```python
from build123d import *

# Parameters (mm, degrees)
SKETCH1_W               = 95.25
SKETCH1_H               = 95.25
BOSS_EXTRUDE1_DEPTH     = 6.35
SKETCH4_W               = 6.35
SKETCH4_H               = 95.25
BOSS_EXTRUDE2_DEPTH     = 12.7
CUT_EXTRUDE1_DEPTH      = 102.649597269
CUT_EXTRUDE1_DEPTH_BACK = 102.649597269
SKETCH5_W               = 22.86
SKETCH5_H               = 12.7
SKETCH6_R               = 1.27
CUT_EXTRUDE2_DEPTH      = 108.247345538
SKETCH7_R               = 1.5875
CUT_EXTRUDE3_DEPTH      = 69.538830235
CUT_EXTRUDE4_DEPTH      = 102.649597269
CUT_EXTRUDE4_DEPTH_BACK = 102.649597269
SKETCH8_R               = 1.5875
SKETCH9_W               = 95.25
SKETCH9_H               = 19.05
BOSS_EXTRUDE3_DEPTH     = 3.175
CUT_EXTRUDE5_DEPTH      = 71.781852371
SKETCH11_W              = 50.8
SKETCH11_H              = 38.1
BOSS_EXTRUDE4_DEPTH     = 4.7625
CUT_EXTRUDE6_REACH      = 115.858
SKETCH12_R              = 1.5875
SKETCH12_W              = 19.05
SKETCH12_H              = 15.875
FILLET1_R               = 6.985
FILLET2_R               = 6.35
FILLET3_R               = 3.175
FILLET4_R               = 3.175
FILLET5_R               = 3.175
SKETCH14_W              = 9.525
SKETCH14_H              = 9.525
BOSS_EXTRUDE5_DEPTH     = 9.525
SKETCH15_R              = 1.905
CUT_EXTRUDE7_DEPTH      = 76.268261904
FILLET7_R               = 1.5875
FILLET8_R               = 1.5875
CUT_EXTRUDE8_START      = -3.175
CUT_EXTRUDE8_DEPTH      = 3.175


with BuildPart() as part:
    # Sketch1 → Boss-Extrude1 (new body)
    with BuildSketch(Plane(origin=(0, 0, 0), x_dir=(1, 0, 0), z_dir=(0, 1, 0))):
        Rectangle(SKETCH1_W, SKETCH1_H)
    extrude(amount=BOSS_EXTRUDE1_DEPTH)

    # Sketch4 → Boss-Extrude2 (add)
    with BuildSketch(Plane(origin=(0, 0, 0), x_dir=(-1, 0, 0), z_dir=(0, -1, 0))):
        with Locations((-44.45, 0)):
            Rectangle(SKETCH4_W, SKETCH4_H)
        with Locations((44.45, 0)):
            Rectangle(SKETCH4_W, SKETCH4_H)
    extrude(amount=BOSS_EXTRUDE2_DEPTH)

    # Sketch5 → Cut-Extrude1 (cut, two sides: drawn at the far end of the back side and taken through both)
    with BuildSketch(Plane(origin=(-41.275, 0, 0), x_dir=(0, 0, -1), z_dir=(1, 0, 0)).offset(-CUT_EXTRUDE1_DEPTH_BACK)):
        with Locations((-22.225, -6.35)):
            Rectangle(SKETCH5_W, SKETCH5_H)
    extrude(amount=CUT_EXTRUDE1_DEPTH + CUT_EXTRUDE1_DEPTH_BACK, mode=Mode.SUBTRACT)

    # Sketch6 → Cut-Extrude2 (cut, through all)
    with BuildSketch(Plane.ZY.offset(47.625)):
        with Locations((36.068, -6.35)):
            Circle(SKETCH6_R)
        with Locations((8.382, -6.35)):
            Circle(SKETCH6_R)
    extrude(amount=-CUT_EXTRUDE2_DEPTH, mode=Mode.SUBTRACT)

    # Sketch7 → Cut-Extrude3 (cut, through all)
    with BuildSketch(Plane.XZ):
        with Locations(Location((27.94, 0, 0), (0, 0, 270))):
            Circle(SKETCH7_R)
        with Locations(Location((-27.94, 0, 0), (0, 0, 270))):
            Circle(SKETCH7_R)
        with Locations(Location((0, 36.83, 0), (0, 0, 270))):
            Circle(SKETCH7_R)
        with Locations(Location((0, -36.83, 0), (0, 0, 270))):
            Circle(SKETCH7_R)
    extrude(amount=-CUT_EXTRUDE3_DEPTH, mode=Mode.SUBTRACT)

    # Sketch8 → Cut-Extrude4 (cut, two sides: drawn at the far end of the back side and taken through both)
    with BuildSketch(Plane(origin=(-41.275, 0, 0), x_dir=(0, 0, -1), z_dir=(1, 0, 0)).offset(-CUT_EXTRUDE4_DEPTH_BACK)):
        with Locations((41.275, -6.35)):
            Circle(SKETCH8_R)
        with Locations((33.3375, -6.35)):
            Circle(SKETCH8_R)
    extrude(amount=CUT_EXTRUDE4_DEPTH + CUT_EXTRUDE4_DEPTH_BACK, mode=Mode.SUBTRACT)

    # Sketch9 → Boss-Extrude3 (add)
    with BuildSketch(Plane.XY.offset(47.625)):
        with Locations((0, -3.175)):
            Rectangle(SKETCH9_W, SKETCH9_H)
    extrude(amount=BOSS_EXTRUDE3_DEPTH)

    # Sketch10 → Cut-Extrude5 (cut, through all)
    with BuildSketch(Plane.XZ):
        with BuildLine():
            Line((-31.75, -38.735), (-35.56, -38.735))
            ThreePointArc((-35.56, -38.735), (-37.356051224, -37.991051224), (-38.1, -36.195))
            Line((-38.1, -36.195), (-38.1, -15.875))
            ThreePointArc((-38.1, -15.875), (-37.356051224, -14.078948776), (-35.56, -13.335))
            Line((-35.56, -13.335), (-31.75, -13.335))
            ThreePointArc((-31.75, -13.335), (-29.953948776, -14.078948776), (-29.21, -15.875))
            Line((-29.21, -15.875), (-29.21, -36.195))
            ThreePointArc((-29.21, -36.195), (-29.953948776, -37.991051224), (-31.75, -38.735))
        make_face()
        with BuildLine():
            Line((35.56, -38.735), (31.75, -38.735))
            ThreePointArc((31.75, -38.735), (29.953948776, -37.991051224), (29.21, -36.195))
            Line((29.21, -36.195), (29.21, -15.875))
            ThreePointArc((29.21, -15.875), (29.953948776, -14.078948776), (31.75, -13.335))
            Line((31.75, -13.335), (35.56, -13.335))
            ThreePointArc((35.56, -13.335), (37.356051224, -14.078948776), (38.1, -15.875))
            Line((38.1, -15.875), (38.1, -36.195))
            ThreePointArc((38.1, -36.195), (37.356051224, -37.991051224), (35.56, -38.735))
        make_face()
    extrude(amount=-CUT_EXTRUDE5_DEPTH, mode=Mode.SUBTRACT)

    # Sketch11 → Boss-Extrude4 (add)
    with BuildSketch(Plane(origin=(0, 0, -47.625), x_dir=(-1, 0, 0), z_dir=(0, 0, -1))):
        with Locations((0, -12.7)):
            Rectangle(SKETCH11_W, SKETCH11_H)
    extrude(amount=-BOSS_EXTRUDE4_DEPTH)

    # Sketch12 → Cut-Extrude6 (cut, up to next)
    with BuildSketch(Plane(origin=(0, 0, -47.625), x_dir=(-1, 0, 0), z_dir=(0, 0, -1)), mode=Mode.PRIVATE) as cut_extrude6_sk1:
        with Locations((-20.701, -8.382)):
            Circle(SKETCH12_R)
    cut_extrude6_tool1 = extrude(cut_extrude6_sk1.sketch, amount=-CUT_EXTRUDE6_REACH, mode=Mode.PRIVATE) & part.part
    # Sketch12 → Cut-Extrude6 (cut, up to next)
    with BuildSketch(Plane(origin=(0, 0, -47.625), x_dir=(-1, 0, 0), z_dir=(0, 0, -1)), mode=Mode.PRIVATE) as cut_extrude6_sk2:
        with Locations((-20.701, -25.4)):
            Circle(SKETCH12_R)
    cut_extrude6_tool2 = extrude(cut_extrude6_sk2.sketch, amount=-CUT_EXTRUDE6_REACH, mode=Mode.PRIVATE) & part.part
    # Sketch12 → Cut-Extrude6 (cut, up to next)
    with BuildSketch(Plane(origin=(0, 0, -47.625), x_dir=(-1, 0, 0), z_dir=(0, 0, -1)), mode=Mode.PRIVATE) as cut_extrude6_sk3:
        with Locations((20.701, -8.382)):
            Circle(SKETCH12_R)
    cut_extrude6_tool3 = extrude(cut_extrude6_sk3.sketch, amount=-CUT_EXTRUDE6_REACH, mode=Mode.PRIVATE) & part.part
    # Sketch12 → Cut-Extrude6 (cut, up to next)
    with BuildSketch(Plane(origin=(0, 0, -47.625), x_dir=(-1, 0, 0), z_dir=(0, 0, -1)), mode=Mode.PRIVATE) as cut_extrude6_sk4:
        with Locations((20.701, -25.4)):
            Circle(SKETCH12_R)
    cut_extrude6_tool4 = extrude(cut_extrude6_sk4.sketch, amount=-CUT_EXTRUDE6_REACH, mode=Mode.PRIVATE) & part.part
    # Sketch12 → Cut-Extrude6 (cut, up to next)
    with BuildSketch(Plane(origin=(0, 0, -47.625), x_dir=(-1, 0, 0), z_dir=(0, 0, -1)), mode=Mode.PRIVATE) as cut_extrude6_sk5:
        with Locations((0, -8.9535)):
            Rectangle(SKETCH12_W, SKETCH12_H)
    cut_extrude6_tool5 = extrude(cut_extrude6_sk5.sketch, amount=-CUT_EXTRUDE6_REACH, mode=Mode.PRIVATE) & part.part
    add(cut_extrude6_tool1.solids().sort_by_distance((20.701, -8.382, -47.625))[0], mode=Mode.SUBTRACT)
    add(cut_extrude6_tool2.solids().sort_by_distance((20.701, -25.4, -47.625))[0], mode=Mode.SUBTRACT)
    add(cut_extrude6_tool3.solids().sort_by_distance((-20.701, -8.382, -47.625))[0], mode=Mode.SUBTRACT)
    add(cut_extrude6_tool4.solids().sort_by_distance((-20.701, -25.4, -47.625))[0], mode=Mode.SUBTRACT)
    add(cut_extrude6_tool5.solids().sort_by_distance((0, -8.9535, -47.625))[0], mode=Mode.SUBTRACT)

    # Fillet1
    fillet1_edges = [part.edges().sort_by_distance(p)[0] for p in [
        (9.525, -1.016, -45.24375),
        (9.525, -16.891, -45.24375),
        (-9.525, -16.891, -45.24375),
        (-9.525, -1.016, -45.24375),
    ]]
    fillet(fillet1_edges, radius=FILLET1_R)

    # Fillet2
    fillet2_edges = [part.edges().sort_by_distance(p)[0] for p in [
        (-25.4, 0, -45.24375),
        (25.4, 0, -45.24375),
    ]]
    fillet(fillet2_edges, radius=FILLET2_R)

    # Fillet3
    fillet3_edges = [part.edges().sort_by_distance(p)[0] for p in [
        (44.45, -12.7, -47.625),
        (-44.45, -12.7, -47.625),
        (44.45, -12.7, 10.795),
        (-44.45, -12.7, 10.795),
        (44.45, -12.7, 33.655),
        (-44.45, -12.7, 33.655),
    ]]
    fillet(fillet3_edges, radius=FILLET3_R)

    # Fillet4
    fillet4_edges = [part.edges().sort_by_distance(p)[0] for p in [
        (41.275, 0, 40.64),
        (41.275, -6.35, 47.625),
        (0, 0, 47.625),
        (-41.275, 0, -18.415),
        (-41.275, -6.35, 47.625),
        (-41.275, 0, 40.64),
        (41.275, 0, -18.415),
    ]]
    fillet(fillet4_edges, radius=FILLET4_R - 0.0001)  # a hair under: the kernel refuses the full size

    # Fillet5
    fillet5_edges = [part.edges().sort_by_distance(p)[0] for p in [
        (-47.625, 6.35, 1.5875),
        (-47.625, -3.175, 50.8),
        (47.625, -3.175, 50.8),
        (0, 6.35, 50.8),
        (47.625, 6.35, 1.5875),
    ]]
    fillet(fillet5_edges, radius=FILLET5_R)

    # Sketch14 → Boss-Extrude5 (add)
    with BuildSketch(Plane.XZ.offset(31.75)):
        with Locations((-30.1625, -42.8625)):
            Rectangle(SKETCH14_W, SKETCH14_H)
        with Locations((30.1625, -42.8625)):
            Rectangle(SKETCH14_W, SKETCH14_H)
    extrude(amount=-BOSS_EXTRUDE5_DEPTH)

    # Sketch15 → Cut-Extrude7 (cut, through all)
    with BuildSketch(Plane(origin=(0, -22.225, 0), x_dir=(1, 0, 0), z_dir=(0, 1, 0))):
        with Locations(Location((-30.1625, 42.8625, 0), (0, 0, 270))):
            Circle(SKETCH15_R)
        with Locations(Location((30.1625, 42.8625, 0), (0, 0, 270))):
            Circle(SKETCH15_R)
    extrude(amount=-CUT_EXTRUDE7_DEPTH, mode=Mode.SUBTRACT)

    # Fillet7
    fillet7_edges = [part.edges().sort_by_distance(p)[0] for p in [
        (-25.4, -26.9875, -42.8625),
        (-25.4, -26.9875, -38.1),
        (-34.925, -26.9875, -47.625),
        (-34.925, -26.9875, -38.1),
        (25.4, -26.9875, -42.8625),
        (25.4, -26.9875, -38.1),
        (34.925, -26.9875, -38.1),
        (34.925, -26.9875, -47.625),
    ]]
    fillet(fillet7_edges, radius=FILLET7_R)

    # Fillet8
    fillet8_edges = [part.edges().sort_by_distance(p)[0] for p in [
        (-25.4, -22.225, -45.24375),
        (25.4, -22.225, -45.24375),
    ]]
    fillet(fillet8_edges, radius=FILLET8_R)

    # Sketch16 → Cut-Extrude8 (cut)
    with BuildSketch(Plane.XZ.offset(31.75).offset(CUT_EXTRUDE8_START)):
        with BuildLine():
            Line((-33.3375, -47.625), (33.3375, -47.625))
            ThreePointArc((33.3375, -47.625), (34.460032015, -47.160032015), (34.925, -46.0375))
            Line((34.925, -46.0375), (34.925, -39.6875))
            ThreePointArc((34.925, -39.6875), (34.460032015, -38.564967985), (33.3375, -38.1))
            Line((33.3375, -38.1), (26.9875, -38.1))
            ThreePointArc((26.9875, -38.1), (25.864967985, -38.564967985), (25.4, -39.6875))
            Line((25.4, -39.6875), (25.4, -41.275))
            ThreePointArc((25.4, -41.275), (24.935032015, -42.397532015), (23.8125, -42.8625))
            Line((23.8125, -42.8625), (-23.8125, -42.8625))
            ThreePointArc((-23.8125, -42.8625), (-24.935032015, -42.397532015), (-25.4, -41.275))
            Line((-25.4, -41.275), (-25.4, -39.6875))
            ThreePointArc((-25.4, -39.6875), (-25.864967985, -38.564967985), (-26.9875, -38.1))
            Line((-26.9875, -38.1), (-33.3375, -38.1))
            ThreePointArc((-33.3375, -38.1), (-34.460032015, -38.564967985), (-34.925, -39.6875))
            Line((-34.925, -39.6875), (-34.925, -46.0375))
            ThreePointArc((-34.925, -46.0375), (-34.460032015, -47.160032015), (-33.3375, -47.625))
        make_face()
    extrude(amount=CUT_EXTRUDE8_DEPTH, mode=Mode.SUBTRACT)


solid = part.part
```
Source: CAD feature listing. Evaluate the final solid. Frame: model axes, mm. A direction names the side the tool comes from. Coordinates: 2 decimals unless noted, no trailing zeros. Write each loop counter-clockwise with the first axis right and the second up, starting at its lowest first coordinate (ties: lowest second). Pieces come first, ordered by that corner, then holes. Notation, with made-up numbers: M 73.25,-11 L 131.25,-11 A18 ccw 131.25,23 Z; hole C 35.25,-27.75 d8. An arc over 180 degrees is marked long. Answer as a JSON object with one key per item and string values.
1. Ray query, L1, parallel to X at y = -8, z = 39 (3 decimals); L2, parallel to Y at x = -11.5, z = 34; L3, parallel to Z at x = -38.5, y = -7.5. Return the intervals inside material, ascending.
Evaluation:
{"L1": "-47.625 to -41.275, 41.275 to 47.625", "L2": "0 to 6.35", "L3": "47.6 to 50.8"}
2. Cut plane B-B on x = 0. State how many separate pieces and enclosed holes the cut face has, plus the area to 3 significant figures.
Evaluation:
{"separate pieces": "4", "enclosed holes": "0", "area": "685 mm^2"}
3. Draft query along Y for faces 1 (the cylindrical face through (-7.533, -3.116, -45.21)), 2 (the flat face through (47.625, -5, -11)), 3 (the cylindrical face through (40.32, -0.905, 38.977)). Return one class per face: released by +Y, released by -Y, zero draft, split by the parting line, or undercut.
Evaluation:
{"face 1": "undercut", "face 2": "zero draft", "face 3": "released by -Y"}
4. Cut plane A-A on y = -25.4. Output: boundary loops of the cut face in (x, z) (1 decimal), plus the area to 3 significant figures.
Evaluation:
{"outline": "M -34.9,-46 A1.6 ccw -33.3,-47.6 L -22.3,-47.6 L -22.3,-42.9 L -23.8,-42.9 A1.6 cw -25.4,-41.3 L -25.4,-39.7 A1.6 ccw -27,-38.1 L -33.3,-38.1 A1.6 ccw -34.9,-39.7 Z; M -19.1,-47.6 L 19.1,-47.6 L 19.1,-42.9 L -19.1,-42.9 Z; M 22.3,-47.6 L 33.3,-47.6 A1.6 ccw 34.9,-46 L 34.9,-39.7 A1.6 ccw 33.3,-38.1 L 27,-38.1 A1.6 ccw 25.4,-39.7 L 25.4,-41.3 A1.6 cw 23.8,-42.9 L 22.3,-42.9 Z; hole C -30.2,-42.9 d3.8; hole C 30.2,-42.9 d3.8", "area": "368 mm^2"}
5. Contact query for flat-ended pins moving along their axis: P1, Ø12, axis at y = -12, z = 30, coming from the -X side (3 decimals); P2, Ø12, axis at x = -15.5, z = 3, coming from the -Y side; P3, Ø0.8, axis at y = -25, z = -40.5, coming from the +X side (3 decimals); P4, Ø7, axis at x = 31, y = -26.5, coming from the +Z side. Output: stop coordinate, or through.
Evaluation:
{"P1": "x = -47.625", "P2": "y = 0", "P3": "x = 34.925", "P4": "z = -38.1"}
6. Access query for faces 4 (the cylindrical face through (-37.336, 3.131, -38.011)), 5 (the cylindrical face through (-29.934, 3.131, -37.971)), 6 (the cylindrical face through (44.494, -11.745, 9.89)), 7 (the cylindrical face through (20.91, -6.81, -45.28)). Directions: +Z, -Z, +X, -X, +Y, -Y. A direction counts if a zero-diameter tool reaches every point of the face in a straight line with its end or side. Return the directions, or none.
Evaluation:
{"face 4": "+Y, -Y", "face 5": "+Y", "face 6": "+X, -X, -Y", "face 7": "-Z"}
